Input: dimensioned drawing with shaded views. Units: mm. Origin: part minimum x, y, z. A direction names the side the tool comes from. Round coordinates to 2 decimals unless told otherwise and drop trailing zeros. Loops run counter-clockwise (first coordinate to the right, second up) from the corner with the lowest first, then second, coordinate; pieces in that order, holes last. Notation, with made-up numbers: (61.5, 29) - (98.5, 29) arc R29 cw to (98.5, 66) - close; hole circle Ø2 at (-24.75, 66.5). An arc over 180 degrees is marked (long way). Answer as CSV lines item,"result".
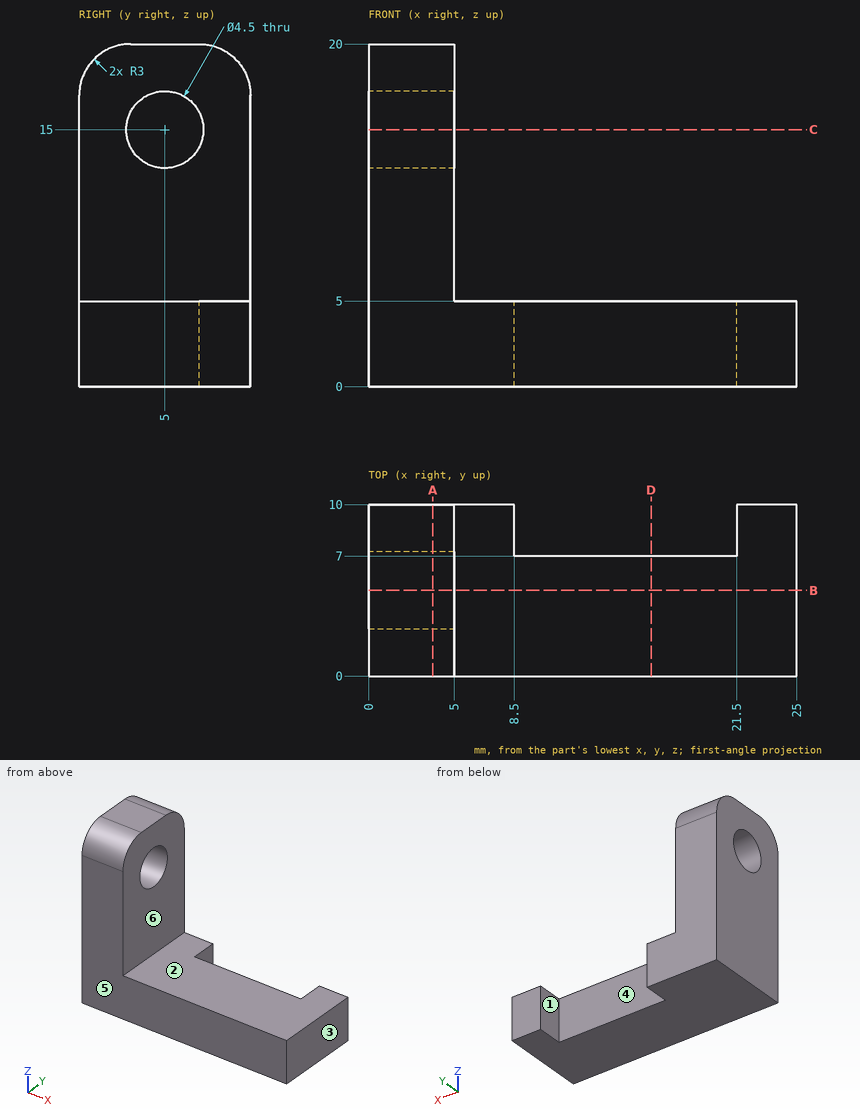
(1) Draft query along X for the marked faces 1, 2 and 3. Return one class per face: pulls with the +X half, pulls with the -X half, needs draft (parallel to the pull), parting line crosses it, or undercut.
Findings below:
face 1,"undercut"
face 2,"needs draft"
face 3,"pulls with the +X half"
(2) Material intervals for line 1 along Z through (x, y) = (1.15, 5); line 2 along X through (y, z) = (8.25, 3.5); line 3 along Z through (x, y) = (21, 4.25), sorted ascending.
Findings below:
line 1,"0 to 12.75, 17.25 to 20"
line 2,"0 to 8.5, 21.5 to 25"
line 3,"0 to 5"
(3) Section C-C (z = 15). Output: boundary loops of the cut face in (x, y), and give its area (3 significant figures).
Findings below:
outline,"(0, 0) - (5, 0) - (5, 2.75) - (0, 2.75) - close; (0, 7.25) - (5, 7.25) - (5, 10) - (0, 10) - close"
area,"27.5 mm2"
(4) Section B-B (y = 5). Output: boundary loops of the cut face in (x, z).
Findings below:
outline,"(0, 0) - (25, 0) - (25, 5) - (5, 5) - (5, 12.75) - (0, 12.75) - close; (0, 17.25) - (5, 17.25) - (5, 20) - (0, 20) - close"
(5) Access query for the marked faces 4, 5 and 6. Directions: +Z, -Z, +X, -X, +Y, -Y. A direction counts if a zero-diameter tool reaches every point of the face in a straight line with its end or side. Return the directions, or none.
Findings below:
face 4,"+Z, -Z, +Y"
face 5,"+Z, -Z, +X, -X, -Y"
face 6,"+Z, +X, +Y, -Y"
(6) Pin query (flat end, axial travel): P1, Ø6, axis at x = 16.5, z = 7, coming from the +Y side; P2, Ø1, axis at x = 14.5, y = 1.5, coming from the +Z side; P3, Ø3, axis at y = 3, z = 11, coming from the +X side. Return the tip coordinate at first contact, or that it passes through.
Findings below:
P1,"y = 7"
P2,"z = 5"
P3,"x = 5"
(7) Section A-A (x = 3.75). Output: boundary loops of the cut face in (y, z), and give its area (3 significant figures).
Findings below:
outline,"(0, 0) - (10, 0) - (10, 17) arc R3 ccw to (7, 20) - (3, 20) arc R3 ccw to (0, 17) - close; hole circle Ø4.5 at (5, 15)"
area,"180 mm2"
(8) Section D-D (x = 16.5). Output: boundary loops of the cut face in (y, z).
Findings below:
outline,"(0, 0) - (7, 0) - (7, 5) - (0, 5) - close"
